Can you work these out from the drawing? Everything is in mm from the part's minimum corner. A direction names the side the tool comes from. Give positions to 0.01 mm unless a question says otherwise; leave off trailing zeros. Loops run counter-clockwise (first coordinate to the right, second up) from the corner with the lowest first, then second, coordinate; pieces in that order, holes last. Notation, with made-up numbers: M 85.5,81.25 L 138.5,81.25 A33 ccw 138.5,119.25 Z; hole C -35.5,83.5 d1. An arc over 180 degrees is marked long. Use CSV: the item, a comma, the result in double quotes.
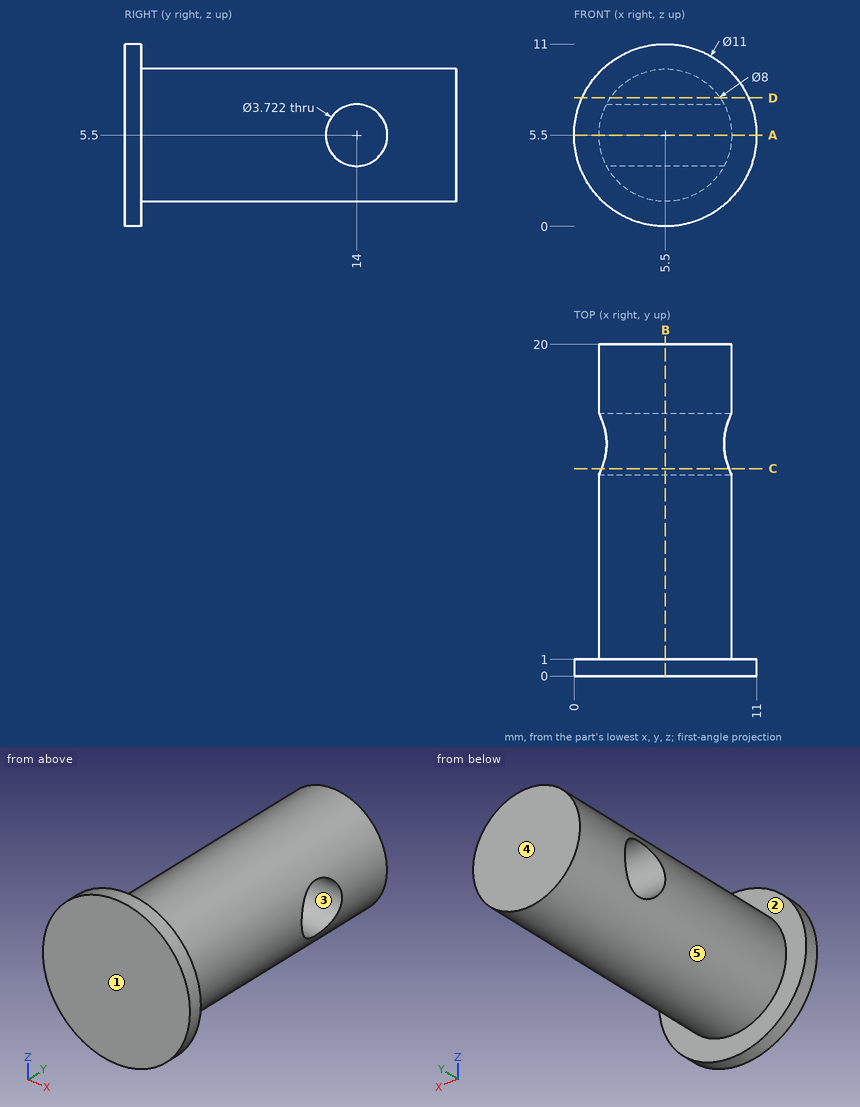
Q1. If we mould it in two halves opening along Y, with no side actions, what happens to the marked faces 1, 2 and 3? For each: released by +Y, released by -Y, zero draft, split by the parting line, or undercut.
Model answer:
face 1,"released by -Y"
face 2,"released by +Y"
face 3,"undercut"
Q2. Please list where these lines run through material, in increasing order: L1, parallel to Y at x = 4.5, z = 5.5; L2, parallel to Y at x = 7.25, z = 1.25; L3, parallel to Z at x = 8, y = 14. Write a range as from..to.
Model answer:
L1,"0..12.14, 15.86..20"
L2,"0..1"
L3,"2.38..3.64, 7.36..8.62"
Q3. I want a section at B-B, the plane x = 5.5. Please give me the cut outline in (y, z), then the cut area to 3 significant figures.
Model answer:
outline,"M 0,0 L 1,0 L 1,1.5 L 20,1.5 L 20,9.5 L 1,9.5 L 1,11 L 0,11 Z; hole C 14,5.5 d3.72"
area,"152 mm2"
Q4. I want a section at D-D, the plane z = 7.75. Please give me the cut outline in (x, y), then the cut area to 3 significant figures.
Model answer:
outline,"M 0.48,0 L 10.52,0 L 10.52,1 L 8.81,1 L 8.81,20 L 2.19,20 L 2.19,1 L 0.48,1 Z"
area,"136 mm2"
Q5. For the marked faces 4 and 5, which set-ups out of +Z, -Z, +X, -X, +Y, -Y let a thin tool reach every point of the face, with its end or its side?
Model answer:
face 4,"+Z, -Z, +X, -X, +Y"
face 5,"+Y"
Q6. I want a section at A-A, the plane z = 5.5. Please give me the cut outline in (x, y), then the cut area to 3 significant figures.
Model answer:
outline,"M 0,0 L 11,0 L 11,1 L 9.5,1 L 9.5,12.14 L 1.5,12.14 L 1.5,1 L 0,1 Z; M 1.5,15.86 L 9.5,15.86 L 9.5,20 L 1.5,20 Z"
area,"133 mm2"
Q7. I'm going to push flat-ended pins straight in: P1, Ø5, axis at x = 8, y = 16, coming from the +Z side; P2, Ø5, axis at y = 5.5, z = 3, coming from the -X side. Where does each tip first touch, or does it pass through?
Model answer:
P1,"z = 9.5"
P2,"x = 1.5"
Q8. I want a section at C-C, the plane y = 12.5. Please give me the cut outline in (x, z) (1 decimal).
Model answer:
outline,"M 1.7,4.4 A4 ccw 9.3,4.4 Z; M 1.7,6.6 L 9.3,6.6 A4 ccw Z"
